Read the model definition and answer for the solid it produces. Units are mm, in the model's axes. Face numbers are marked on the shaded views. A direction names the side the tool comes from. Coordinates: 2 decimals unless noted, no trailing zeros. Write each loop counter-clockwise with the first axis right and the second up, starting at its lowest first coordinate (ties: lowest second). Pieces come first, ordered by that corner, then holes.
(1) Which of the six approach directions +Z, -Z, +X, -X, +Y, -Y give full straight-line access (tool end or side, diameter ignored) to the marked faces 4, 5 and 6?
(2) Determine the mould class of the marked faces 1, 2 and 3 for opening direction Y: pulls with the +Y half, pulls with the -Y half, needs draft (parallel to the pull), parting line crosses it, or undercut.
(3) The part is cut by section C-C, the plane z = -6.5. Determine the outline of the cut face in (x, y).
(4) The part is cut by section B-B, the plane x = 18. Determine the outline of the cut face in (y, z).
(5) Given pin 1 (10 mm diameter, centred on x = 13.5, z = -244, fed in from -Y); pin 2 (1.5 mm diameter, centred on x = -1, y = -331, fed in from -Z); pin 3 (4 mm diameter, centred on x = 65.5, z = -102.5, fed in from +Y), each flat-ended and moving along its own axis, determine where each tip first touches the part or whether it passes through.
(6) The part is cut by section A-A, the plane y = -196. Determine the outline of the cut face in (x, z), and give its area (3 significant figures).
(7) The part is cut by section D-D, the plane z = -176. State how many separate pieces and enclosed holes the cut face has, and give its area (3 significant figures).
(8) Straight lines are drawn through the part: line 1 along Y through (x, z) = (52, -308.5); line 2 along X through (y, z) = (-330, -344.75); line 3 along X through (y, z) = (-310.5, -145.5). For each, find the intervals that lie inside material, in ascending order.
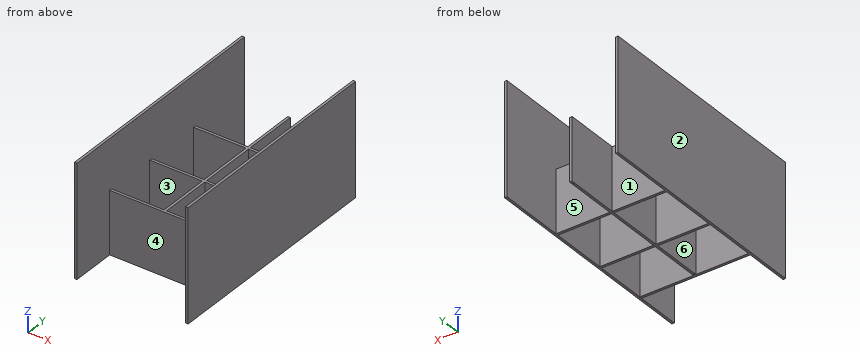
```python
from build123d import *

# Parameters (mm, degrees)
CROQUIS1_W              = 500
CROQUIS1_H              = 690
SALIENTE_EXTRUIR1_DEPTH = 350
CROQUIS2_W              = 245
CROQUIS2_H              = 210
CROQUIS2_H_2            = 230
CROQUIS2_H_3            = 220
CORTAR_EXTRUIR5_DEPTH   = 552.38462075
CROQUIS6_R              = 2.5
CORTAR_EXTRUIR6_DEPTH   = 10
CROQUIS8_W              = 454.743369925
CROQUIS8_H              = 727.77201974
CORTAR_EXTRUIR7_DEPTH   = 100
CROQUIS10_W             = 10
CROQUIS10_H             = 230
CROQUIS10_H_2           = 210
CROQUIS10_H_3           = 220
SALIENTE_EXTRUIR2_DEPTH = 250
CROQUIS11_W             = 564.486110896
CROQUIS11_H             = 131.072073745
CORTAR_EXTRUIR8_DEPTH   = 638.102817448
CROQUIS12_W             = 20.345466795
CROQUIS12_H             = 250
CROQUIS12_W_2           = 24.91116328
CORTAR_EXTRUIR9_DEPTH   = 638.102817448
CROQUIS13_W             = 10
CROQUIS13_H             = 920
SALIENTE_EXTRUIR3_DEPTH = 250
CROQUIS15_W             = 10
CROQUIS15_H             = 920
SALIENTE_EXTRUIR4_DEPTH = 200


with BuildPart() as part:
    # Croquis1 → Saliente-Extruir1 (new body)
    with BuildSketch(Plane.XY):
        Rectangle(CROQUIS1_W, CROQUIS1_H)
    extrude(amount=-SALIENTE_EXTRUIR1_DEPTH)

    # Croquis2 → Cortar-Extruir5 (cut, through all)
    with BuildSketch(Plane.XY):
        with Locations((127.5, -230)):
            Rectangle(CROQUIS2_W, CROQUIS2_H)
        with Locations((-127.5, -230)):
            Rectangle(CROQUIS2_W, CROQUIS2_H)
        with Locations((127.5, 0)):
            Rectangle(CROQUIS2_W, CROQUIS2_H_2)
        with Locations((-127.5, 0)):
            Rectangle(CROQUIS2_W, CROQUIS2_H_2)
        with Locations((127.5, 235)):
            Rectangle(CROQUIS2_W, CROQUIS2_H_3)
        with Locations((-127.5, 235)):
            Rectangle(CROQUIS2_W, CROQUIS2_H_3)
    extrude(amount=-CORTAR_EXTRUIR5_DEPTH, mode=Mode.SUBTRACT)

    # Croquis6 → Cortar-Extruir6 (cut)
    with BuildSketch(Plane(origin=(0, 0, -350), x_dir=(-1, 0, 0), z_dir=(0, 0, -1))):
        with Locations((0, 330)):
            Circle(CROQUIS6_R)
        with Locations(Location((0, -330, 0), (0, 0, 180))):
            Circle(CROQUIS6_R)
    extrude(amount=-CORTAR_EXTRUIR6_DEPTH, mode=Mode.SUBTRACT)

    # Croquis8 → Cortar-Extruir7 (cut)
    with BuildSketch(Plane.XY):
        with Locations((2.282848242, -2.282848243)):
            Rectangle(CROQUIS8_W, CROQUIS8_H)
    extrude(amount=-CORTAR_EXTRUIR7_DEPTH, mode=Mode.SUBTRACT)

    # Croquis10 → Saliente-Extruir2 (add)
    with BuildSketch(Plane.XY.offset(-100)):
        Polygon((219.654533205, 345.243801015), (219.654533205, 125), (229.654533205, 125), (229.654533205, 345.045421076), align=None)
        with Locations((224.654533205, 0)):
            Rectangle(CROQUIS10_W, CROQUIS10_H)
        with Locations((224.654533205, -230)):
            Rectangle(CROQUIS10_W, CROQUIS10_H_2)
        with Locations((-220.08883672, -230)):
            Rectangle(CROQUIS10_W, CROQUIS10_H_2)
        with Locations((-220.08883672, 0)):
            Rectangle(CROQUIS10_W, CROQUIS10_H)
        with Locations((-220.08883672, 235)):
            Rectangle(CROQUIS10_W, CROQUIS10_H_3)
    extrude(amount=-SALIENTE_EXTRUIR2_DEPTH)

    # Croquis11 → Cortar-Extruir8 (cut, through all)
    with BuildSketch(Plane(origin=(0, 125, 0), x_dir=(1, 0, 0), z_dir=(0, 1, 0))):
        with Locations((-2.812204357, 34.463963128)):
            Rectangle(CROQUIS11_W, CROQUIS11_H)
    extrude(amount=-CORTAR_EXTRUIR8_DEPTH, mode=Mode.SUBTRACT)

    # Croquis12 → Cortar-Extruir9 (cut, through all)
    with BuildSketch(Plane(origin=(0, 125, 0), x_dir=(1, 0, 0), z_dir=(0, 1, 0))):
        with Locations((239.827266603, 225)):
            Rectangle(CROQUIS12_W, CROQUIS12_H)
        with Locations((-237.54441836, 225)):
            Rectangle(CROQUIS12_W_2, CROQUIS12_H)
    extrude(amount=-CORTAR_EXTRUIR9_DEPTH, mode=Mode.SUBTRACT)

    # Croquis13 → Saliente-Extruir3 (add)
    with BuildSketch(Plane.XY.offset(-100)):
        with Locations((224.654533205, -65)):
            Rectangle(CROQUIS13_W, CROQUIS13_H)
        with Locations((-220.08883672, -65)):
            Rectangle(CROQUIS13_W, CROQUIS13_H)
    extrude(amount=-SALIENTE_EXTRUIR3_DEPTH)

    # Croquis15 → Saliente-Extruir4 (add)
    with BuildSketch(Plane.XY.offset(-100)):
        with Locations((224.654533205, -65)):
            Rectangle(CROQUIS15_W, CROQUIS15_H)
        with Locations((-220.08883672, -65)):
            Rectangle(CROQUIS15_W, CROQUIS15_H)
    extrude(amount=SALIENTE_EXTRUIR4_DEPTH)


solid = part.part
```
Computed:
1. face 4: +Z, -Z, -Y
1. face 5: +Z, -Z, +Y
1. face 6: +Z, -Z
2. face 1: pulls with the +Y half
2. face 2: needs draft
2. face 3: undercut
3. outline: (-225.09, -525) - (-215.09, -525) - (-215.09, 395) - (-225.09, 395) - close; (219.65, -525) - (229.65, -525) - (229.65, 395) - (219.65, 395) - close
4. outline: (-345, -350) - (-335, -350) - (-335, -100) - (-345, -100) - close; (-125, -350) - (-115, -350) - (-115, -100) - (-125, -100) - close; (115, -350) - (125, -350) - (125, -100) - (115, -100) - close
5. pin 1: stops at y = -345
5. pin 2: stops at z = -340
5. pin 3: stops at y = 125
6. outline: (-225.09, -350) - (-215.09, -350) - (-215.09, 100) - (-225.09, 100) - close; (-5, -350) - (5, -350) - (5, -100) - (-5, -100) - close; (219.65, -350) - (229.65, -350) - (229.65, 100) - (219.65, 100) - close
6. area: 11,500 mm2
7. separate pieces: 1
7. enclosed holes: 4
7. area: 38,000 mm2
8. line 1: y = -345 to -335, -125 to -115, 115 to 125
8. line 2: x = -225.09 to -215.09, -5 to -2.5, 2.5 to 5, 219.65 to 229.65
8. line 3: x = -225.09 to -215.09, -5 to 5, 219.65 to 229.65
